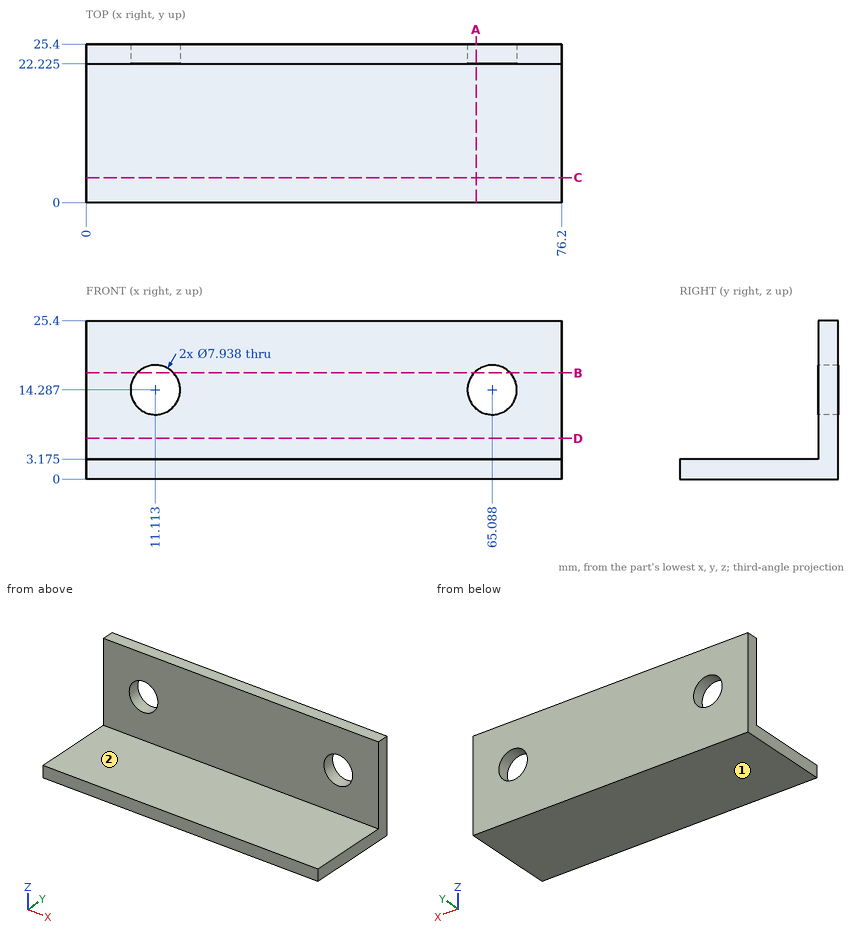
Input: dimensioned drawing with shaded views. Units: mm. Origin: part minimum x, y, z. A direction names the side the tool comes from. Give positions to 0.01 mm unless a question says otherwise; leave off trailing zeros. Write each loop counter-clockwise with the first axis right and the second up, starting at its lowest first coordinate (ties: lowest second). Pieces come first, ordered by that corner, then holes.
1. Section query D-D, the plane z = 6.5. Return loops of the section in (x, y) (1 decimal), then the cut area to 3 significant figures.
2. Section query B-B, the plane z = 17. Return loops of the section in (x, y) (1 decimal).
3. Section query C-C, the plane y = 4. Return loops of the section in (x, z) (1 decimal), then the cut area to 3 significant figures.
4. Section query A-A, the plane x = 62.5. Return loops of the section in (y, z) (1 decimal).
5. Reachability of the marked faces 1 and 2 from +Z, -Z, +X, -X, +Y, -Y: full face, straight path, thin tool, end or side. Return the list, or none.
6. Line query: probe 1 along X at (y, z) = (24.25, 11.75) (1 decimal); probe 2 along Z at (x, y) = (29.5, 17.25) (1 decimal); probe 3 along Y at (x, z) = (41.5, 16.25) (1 decimal). Output: solid intervals per line, ascending.
7. Pin query (flat end, axial travel): P1, Ø5, axis at x = 27, y = 8.5, coming from the +Z side (1 decimal); P2, Ø5, axis at x = 11, y = 17, coming from the -Z side; P3, Ø5, axis at y = 7.5, z = 7.5, coming from the -X side; P4, Ø10.5, axis at x = 11.11, z = 14.29, coming from the -Y side (1 decimal). Return the tip coordinate at first contact, or that it passes through.
Computed:
1. outline: (0, 22.2) - (76.2, 22.2) - (76.2, 25.4) - (0, 25.4) - close
1. area: 242 mm2
2. outline: (0, 22.2) - (8.2, 22.2) - (8.2, 25.4) - (0, 25.4) - close; (14, 22.2) - (62.2, 22.2) - (62.2, 25.4) - (14, 25.4) - close; (68, 22.2) - (76.2, 22.2) - (76.2, 25.4) - (68, 25.4) - close
3. outline: (0, 0) - (76.2, 0) - (76.2, 3.2) - (0, 3.2) - close
3. area: 242 mm2
4. outline: (0, 0) - (25.4, 0) - (25.4, 11.3) - (22.2, 11.3) - (22.2, 3.2) - (0, 3.2) - close; (22.2, 17.3) - (25.4, 17.3) - (25.4, 25.4) - (22.2, 25.4) - close
5. face 1: -Z, +X, -X, +Y, -Y
5. face 2: +Z, +X, -X, -Y
6. probe 1: x = 0 to 8.1, 14.2 to 62, 68.1 to 76.2
6. probe 2: z = 0 to 3.2
6. probe 3: y = 22.2 to 25.4
7. P1: stops at z = 3.2
7. P2: stops at z = 0
7. P3: passes through
7. P4: stops at y = 22.2
